```python
from build123d import *

# Parameters (mm, degrees)
F0_R     = 7.5
F0_R_2   = 10
F1_DEPTH = 20
F2_R     = 20
F3_T     = -8
F4_R     = 2
F6_SIZE  = 1


# Not quite as in the source:
# - two fillets or chamfers of one size are made in one step


with BuildPart() as f1:
    # F0 (on Top) → F1 (new body)
    with BuildSketch(Plane.XY):
        with BuildLine():
            Line((-18.6164580262, 7.8960385923), (-33.8581929877, -28.9007646659))
            ThreePointArc((-33.8581929877, -28.9007646659), (-27.5, -47.6313972081), (-8.0996998956, -43.7724375865))
            Line((-8.0996998956, -43.7724375865), (10.6191461494, -19.3775624703))
            Line((10.6191461494, -19.3775624703), (61.3073361412, -14.9429204714))
            ThreePointArc((61.3073361412, -14.9429204714), (75, 0), (61.3073361412, 14.9429204714))
            Line((61.3073361412, 14.9429204714), (1.604247479, 20.1662639068))
            ThreePointArc((1.604247479, 20.1662639068), (-10.5143325391, 17.3406073584), (-18.6164580262, 7.8960385923))
        make_face()
        with Locations((-20, -34.6410161514)):
            Circle(F0_R, mode=Mode.SUBTRACT)
        Circle(F0_R_2, mode=Mode.SUBTRACT)
        with Locations((60, 0)):
            Circle(F0_R, mode=Mode.SUBTRACT)
    extrude(amount=F1_DEPTH)

    # F2
    f2_edges = [f1.edges().sort_by_distance(p)[0] for p in [
        (10.619146, -19.377562, 10),
    ]]
    fillet(f2_edges, radius=F2_R)

    # F3
    f3_openings = [f1.faces().sort_by_distance(p)[0] for p in [
        (14.636401, -7.453279, 20),
    ]]
    offset(amount=F3_T, openings=f3_openings)

    # F4
    f4_edges = [f1.edges().sort_by_distance(p)[0] for p in [
        (-6.027772, -27.930812, 14),
        (13.849674, -11.497241, 14),
        (2.246879, -17.859214, 14),
        (46.833398, -8.178667, 14),
        (-21.174906, -19.185609, 14),
        (-16.348079, -7.532617, 14),
        (14.22329, 11.031682, 14),
        (46.833398, 8.178667, 14),
    ]]
    fillet(f4_edges, radius=F4_R)

    # F6
    f6_edges = [f1.edges().sort_by_distance(p)[0] for p in [
        (40.346603, -16.776747, 20),
        (-10, 0, 20),
        (31.29601, -9.538013, 20),
        (31.044956, 9.559977, 20),
        (17.546547, -4.014808, 20),
        (17.547047, 4.012624, 20),
        (-8.997951, -15.58964, 20),
        (44.5, 0, 20),
        (-27.5, -34.641016, 20),
        (-12.25, -21.217622, 20),
        (-2.661098, -23.543277, 20),
        (-18.959422, -13.836957, 20),
        (52.5, 0, 20),
        (18.453201, -10.662615, 20),
        (16.373656, -9.84693, 20),
        (45.430722, -7.49354, 20),
        (16.366311, 9.828794, 20),
        (45.430722, 7.49354, 20),
        (-1.418891, -35.065838, 20),
        (11.509209, -20.999932, 20),
        (75, 0, 20),
        (31.455792, 17.554592, 20),
        (-10.514333, 17.340607, 20),
        (-26.237326, -10.502363, 20),
        (-27.5, -47.631397, 20),
        (-0.936161, -21.297027, 20),
        (-0.501696, -19.09992, 20),
        (-5.851945, -26.379688, 20),
        (-16.270071, -9.986458, 20),
        (-19.919507, -18.257777, 20),
    ]]
    chamfer(f6_edges, length=F6_SIZE)


solid = f1.part
```
Verification items for the finished model (mm, model axes). A direction names the side the tool comes from. Round coordinates to 2 decimals unless told otherwise and drop trailing zeros. Order: outer loops, then holes, each group sorted by start corner. A loop starts at its lowest first (then second) coordinate and runs counter-clockwise, first axis right, second up. Notation, with made-up numbers: (4.25, -11) -> (53.25, -11) arc R24 cw to (53.25, 2) -> close; hole circle Ø3 at (11, 42). An arc over 180 degrees is marked (long way). Put each result on its own line as item: value. Start each with the question number.
(1) Section check B-B (y = 0). Enter the section's corners in (x, z).
(2) Tool access check on faces 4 (the face through (11.33, -20.917, 19.16)), 5 (the face through (18, 0, 13)). Record the directions out of +Z, -Z, +X, -X, +Y, -Y that give a thin tool (end or side, any length) a straight path to the whole face; none if there is none.
(3) Section check C-C (z = 5). Enter the section's corners in (x, y).
(4) Depth check by flat-ended pin: pin 1 Ø18 at (x, y) = (0, 0) entering from -Z; pin 2 Ø3 at (y, z) = (12, 6.5) entering from +X; pin 3 Ø12 at (x, z) = (38, 13) entering from -Y; pin 4 Ø1.5 at (x, z) = (37, 17) entering from +Y. Enter the tip coordinate at first touch or a pass-through.
(5) Section check A-A (x = 60). Enter the section's corners in (y, z), then the cut area to 3 significant figures.
(6) Material ranges on line 1 along X through (y, z) = (-0.5, 11); line 2 along X through (y, z) = (-0.5, 5.25); line 3 along Y through (x, z) = (-16, 14.5), recorded low to high.
(7) Draft check along Y on faces 1 (the face through (75, 0, 9)), 2 (the face through (-1.512, -35.188, 9.367)), 3 (the face through (-18.944, -13.8, 13.423)). Enter one of: +Y half, -Y half, draft (parallel to the pull), parting line (faces both ways), or undercut.
Completed:
1. outline: (-21.89, 0) -> (-10, 0) -> (-10, 19) -> (-11, 20) -> (-20.8, 20) -> (-21.89, 19) -> close; (10, 0) -> (52.5, 0) -> (52.5, 19) -> (51.5, 20) -> (45.5, 20) -> (44.5, 19) -> (44.5, 8) -> (18, 8) -> (18, 19) -> (17, 20) -> (11, 20) -> (10, 19) -> close; (67.5, 0) -> (75, 0) -> (75, 19) -> (74, 20) -> (68.5, 20) -> (67.5, 19) -> close
2. face 4: +Z, +X, -Y
2. face 5: +Z
3. outline: (-33.86, -28.9) arc R15 ccw to (-8.1, -43.77) -> (5.26, -26.36) arc R20 cw to (19.39, -18.61) -> (61.31, -14.94) arc R15 ccw to (61.31, 14.94) -> (1.6, 20.17) arc R20 ccw to (-18.62, 7.9) -> close; hole circle Ø15 at (-20, -34.64); hole circle Ø20 at (0, 0); hole circle Ø15 at (60, 0)
4. pin 1: passes through
4. pin 2: stops at x = 70.71
4. pin 3: stops at y = -17.51
4. pin 4: stops at y = 17.14
5. outline: (-15.06, 0) -> (-7.5, 0) -> (-7.5, 19) -> (-8.5, 20) -> (-14.05, 20) -> (-15.06, 19) -> close; (7.5, 0) -> (15.06, 0) -> (15.06, 19) -> (14.05, 20) -> (8.5, 20) -> (7.5, 19) -> close
5. area: 300 mm2
6. line 1: x = -22.09 to -9.99, 9.99 to 17.99, 44.51 to 52.52, 67.48 to 74.99
6. line 2: x = -22.09 to -9.99, 9.99 to 52.52, 67.48 to 74.99
6. line 3: y = -49.1 to -40.99, -28.3 to -19.67, -9.97 to 12.43
7. face 1: parting line
7. face 2: -Y half
7. face 3: undercut
